```python
from build123d import *

# Parameters (mm, degrees)
F0_W     = 101.6
F0_H     = 50.8
F1_DEPTH = 25.4
F2_R     = 6.35
F3_DEPTH = 25.401
F4_W     = 12.7
F4_H     = 50.8
F6_W     = 11.6320042121
F6_H     = 12.7
F8_R     = 2.54
F9_SIZE  = 2.54


with BuildPart() as f1:
    # F0 (on Top) → F1 (new body)
    with BuildSketch(Plane.XY):
        Rectangle(F0_W, F0_H)
    extrude(amount=F1_DEPTH)

    # F2 (on face) → F3 (cut, through all)
    with BuildSketch(Plane.XY.offset(25.4)):
        with Locations((-38.1, 12.7)):
            Circle(F2_R)
        with Locations((-38.1, -12.7)):
            Circle(F2_R)
        with Locations((38.1, -12.7)):
            Circle(F2_R)
        with Locations((38.1, 12.7)):
            Circle(F2_R)
    extrude(amount=-F3_DEPTH, mode=Mode.SUBTRACT)

    # F4 (on Front) → F5 (revolve)
    with BuildSketch(Plane.XZ):
        with Locations((-6.35, 50.8)):
            Rectangle(F4_W, F4_H)
    revolve(axis=Axis((0, 0, 50.8), (0, 0, 1)))

    # F6 (on Front) → F7 (revolve, cut)
    with BuildSketch(Plane.XZ):
        with Locations((12.166002106, 57.15)):
            Rectangle(F6_W, F6_H)
    revolve(axis=Axis((0, 0, 43.5032770038), (0, 0, 1)), mode=Mode.SUBTRACT)

    # F8
    f8_edges = [f1.edges().sort_by_distance(p)[0] for p in [
        (12.7, 0, 50.8),
        (-6.35, 0, 63.5),
        (12.7, 0, 63.5),
        (12.7, 0, 25.4),
        (12.7, 0, 76.2),
    ]]
    fillet(f8_edges, radius=F8_R)

    # F9
    f9_edges = [f1.edges().sort_by_distance(p)[0] for p in [
        (0, -25.4, 25.4),
        (-50.8, 0, 25.4),
        (0, 25.4, 25.4),
        (50.8, 0, 25.4),
    ]]
    chamfer(f9_edges, length=F9_SIZE)


solid = f1.part
```
For this review, take the finished solid that the model builds, in its own axes (mm). A direction names the side the tool comes from. Give positions to 0.01 mm unless a question says otherwise; leave off trailing zeros. Loops run counter-clockwise (first coordinate to the right, second up) from the corner with the lowest first, then second, coordinate; pieces in that order, holes last. Notation, with made-up numbers: M 25,-0.5 L 41,-0.5 A27 ccw 41,15.5 Z; hole C 12.5,81.25 d5. An arc over 180 degrees is marked long. One line per item, written item: value. Start each with the question number.
Q1. Add section B-B (z = 19.5). Give the boundary of the cut face in (x, y).
Q2. Add section D-D (y = 0). Give the boundary of the cut face in (x, z).
Q3. Add section A-A (x = 38.1). Give the boundary of the cut face in (y, z).
Q4. For L1, parallel to Y at x = -38, z = 14; L2, parallel to Z at x = -22, y = -13; L3, parallel to X at y = -12, z = 12, list the stretches that pass through material, from the lowest coordinate up.
Q5. Clearance check with flat-ended pins moving along their axes: pin 1 Ø16.5 at (x, y) = (38.1, 12.7) entering from +Z; pin 2 Ø4 at (x, z) = (1.5, 39) entering from -Y; pin 3 Ø3 at (x, z) = (-10.5, 50.5) entering from +Y. State where each tip first meets the part, or that it passes through.
Q6. Draft analysis for pull direction Z (two halves, no side actions). For faces 4 (the face through (-1, 0, 0)), 5 (the face through (31.756, -12.421, 12.878)), 6 (the face through (0, -7, 50.8)), state which applies: released by +Z, released by -Z, zero draft, split by the parting line, or undercut.
Q7. Machinability: for faces 1 (the face through (2.75, 12.4, 38.24)), 2 (the face through (50.8, 0, 11)), 3 (the face through (-1, -9, 63.5)), which of the approach directions +Z, -Z, +X, -X, +Y, -Y give a long, thin tool a straight path to every point of the face, cutting with its end or side? Answer none if there is none.
Q8. Add section C-C (x = 0). Give the boundary of the cut face in (y, z), and give its area (3 significant figures).
Reply:
1. outline: M -50.8,-25.4 L 50.8,-25.4 L 50.8,25.4 L -50.8,25.4 Z; hole C -38.1,-12.7 d12.7; hole C -38.1,12.7 d12.7; hole C 38.1,-12.7 d12.7; hole C 38.1,12.7 d12.7
2. outline: M -50.8,0 L 50.8,0 L 50.8,22.86 L 48.26,25.4 L 15.24,25.4 A2.54 cw 12.7,27.94 L 12.7,48.26 A2.54 ccw 10.16,50.8 L 6.35,50.8 L 6.35,60.96 A2.54 cw 8.89,63.5 L 10.16,63.5 A2.54 ccw 12.7,66.04 L 12.7,73.66 A2.54 ccw 10.16,76.2 L -10.16,76.2 A2.54 ccw -12.7,73.66 L -12.7,66.04 A2.54 ccw -10.16,63.5 L -8.89,63.5 A2.54 cw -6.35,60.96 L -6.35,50.8 L -10.16,50.8 A2.54 ccw -12.7,48.26 L -12.7,27.94 A2.54 cw -15.24,25.4 L -48.26,25.4 L -50.8,22.86 Z
3. outline: M -25.4,0 L -19.05,0 L -19.05,25.4 L -22.86,25.4 L -25.4,22.86 Z; M -6.35,0 L 6.35,0 L 6.35,25.4 L -6.35,25.4 Z; M 19.05,0 L 25.4,0 L 25.4,22.86 L 22.86,25.4 L 19.05,25.4 Z
4. L1: -25.4 to -19.05, -6.35 to 6.35, 19.05 to 25.4
4. L2: 0 to 25.4
4. L3: -50.8 to -44.41, -31.79 to 31.79, 44.41 to 50.8
5. pin 1: z = 25.4
5. pin 2: y = -12.7
5. pin 3: y = 8.08
6. face 4: released by -Z
6. face 5: zero draft
6. face 6: undercut
7. face 1: +Z
7. face 2: +Z, -Z, +X, +Y, -Y
7. face 3: none
8. outline: M -25.4,0 L 25.4,0 L 25.4,22.86 L 22.86,25.4 L 15.24,25.4 A2.54 cw 12.7,27.94 L 12.7,48.26 A2.54 ccw 10.16,50.8 L 6.35,50.8 L 6.35,60.96 A2.54 cw 8.89,63.5 L 10.16,63.5 A2.54 ccw 12.7,66.04 L 12.7,73.66 A2.54 ccw 10.16,76.2 L -10.16,76.2 A2.54 ccw -12.7,73.66 L -12.7,66.04 A2.54 ccw -10.16,63.5 L -8.89,63.5 A2.54 cw -6.35,60.96 L -6.35,50.8 L -10.16,50.8 A2.54 ccw -12.7,48.26 L -12.7,27.94 A2.54 cw -15.24,25.4 L -22.86,25.4 L -25.4,22.86 Z
8. area: 2,410 mm²
